Read the model definition and answer for the solid it produces. Units are mm, in the model's axes. A direction names the side the tool comes from. Coordinates: 2 decimals unless noted, no trailing zeros. Write each loop counter-clockwise with the first axis right and the second up, starting at its lowest first coordinate (ties: lowest second). Pieces come first, ordered by that corner, then holes. Notation, with made-up numbers: (80.5, 2.25) -> (87.5, 2.25) arc R35 ccw to (87.5, 36.25) -> close; hole circle Ø3 at (-10.5, 68). An arc over 180 degrees is marked (long way). Answer as a JSON object with one key per item and string values. Group by question number.
(1) Straight lines are drawn through the part: L1, parallel to Y at x = 0, z = 7.05; L2, parallel to X at y = 3, z = 6.75; L3, parallel to Z at x = 4.25, y = 3.75. For each, find the intervals that lie inside material, in ascending order.
(2) Find section D-D (z = 8.25). Give the vertices of the cut face in (x, y).
(3) Find section A-A (y = 0). Give the vertices of the cut face in (x, z).
(4) Find section C-C (z = 7.4). Give the vertices of the cut face in (x, y).
(5) Flat-ended cylindrical pins translate along their axes: P1, Ø2, axis at x = -4.33, y = 2.5, coming from the -Z side; P2, Ø1.8, axis at x = 0, y = 5, coming from the +Z side. Find the tip coordinate at first contact, or state that the pin passes through.
(6) Find section B-B (x = 0). Give the vertices of the cut face in (y, z).
(7) Which of the six approach directions +Z, -Z, +X, -X, +Y, -Y give full straight-line access (tool end or side, diameter ignored) to faces 4 (the face through (-0.878, -3.956, 8.364)), 5 (the face through (0.312, -5.597, 7.147))?
(8) For a pull along Y with two mould halves and no side action, classify faces 1 (the face through (2.805, -5.392, 7.013)), 2 (the face through (-1, 3, 9.182)), 3 (the face through (-3.684, 2.702, 7.147)) as +Y half, -Y half, draft (parallel to the pull), parting line (faces both ways), or undercut.
from build123d import *

# Parameters (mm, degrees)
SKETCH1_R           = 45
SKETCH1_R_2         = 30
SKETCH1_R_3         = 5
BOSS_EXTRUDE1_DEPTH = 10
SKETCH1_3_R         = 30
SKETCH1_3_R_2       = 20
BOSS_EXTRUDE2_DEPTH = 20
FILLET1_R           = 2
SCALE_1_SCALE       = 0.135064935


with BuildPart() as part:
    # Sketch1 → Boss-Extrude1 (new body)
    with BuildSketch(Plane.XY):
        Circle(SKETCH1_R)
        Circle(SKETCH1_R_2, mode=Mode.SUBTRACT)
        with Locations((-32.04293994, 18.5)):
            Circle(SKETCH1_R_3, mode=Mode.SUBTRACT)
        with Locations((-32.04293994, -18.5)):
            Circle(SKETCH1_R_3, mode=Mode.SUBTRACT)
        with Locations((0, -37)):
            Circle(SKETCH1_R_3, mode=Mode.SUBTRACT)
        with Locations((32.04293994, -18.5)):
            Circle(SKETCH1_R_3, mode=Mode.SUBTRACT)
        with Locations((32.04293994, 18.5)):
            Circle(SKETCH1_R_3, mode=Mode.SUBTRACT)
        with Locations((0, 37)):
            Circle(SKETCH1_R_3, mode=Mode.SUBTRACT)
    extrude(amount=BOSS_EXTRUDE1_DEPTH)

    # Sketch1_3 → Boss-Extrude2 (add)
    with BuildSketch(Plane.XY):
        Circle(SKETCH1_3_R)
        Circle(SKETCH1_3_R_2, mode=Mode.SUBTRACT)
    extrude(amount=BOSS_EXTRUDE2_DEPTH)

    # Fillet1
    fillet1_edges = [part.edges().sort_by_distance(p)[0] for p in [
        (-30, 0, 20),
        (-45, 0, 10),
    ]]
    fillet(fillet1_edges, radius=FILLET1_R)


with BuildPart() as part_1:
    # Scale 1: scaled about (0, 0, 7.492696154)
    add(part.part.scale(SCALE_1_SCALE).moved(Location((0, 0, 6.480695634))))


solid = part_1.part
Results below:
{
 "1": {"L1": "y = -6.08 to -5.67, -4.32 to -2.7, 2.7 to 4.32, 5.67 to 6.08", "L2": "x = -5.29 to -4.78, -3.88 to 3.88, 4.78 to 5.29", "L3": "z = 6.48 to 7.83"},
 "2": {"outline": "circle Ø8.1 at (0, 0); hole circle Ø5.4 at (0, 0)"},
 "3": {"outline": "(-6.08, 6.48) -> (-2.7, 6.48) -> (-2.7, 9.18) -> (-3.78, 9.18) arc R0.27 ccw to (-4.05, 8.91) -> (-4.05, 7.83) -> (-5.81, 7.83) arc R0.27 ccw to (-6.08, 7.56) -> close; (2.7, 6.48) -> (6.08, 6.48) -> (6.08, 7.56) arc R0.27 ccw to (5.81, 7.83) -> (4.05, 7.83) -> (4.05, 8.91) arc R0.27 ccw to (3.78, 9.18) -> (2.7, 9.18) -> close"},
 "4": {"outline": "circle Ø12.16 at (0, 0); hole circle Ø1.35 at (-4.33, -2.5); hole circle Ø1.35 at (-4.33, 2.5); hole circle Ø5.4 at (0, 0); hole circle Ø1.35 at (0, -5); hole circle Ø1.35 at (0, 5); hole circle Ø1.35 at (4.33, -2.5); hole circle Ø1.35 at (4.33, 2.5)"},
 "5": {"P1": "stops at z = 6.48", "P2": "stops at z = 7.83"},
 "6": {"outline": "(-6.08, 6.48) -> (-5.67, 6.48) -> (-5.67, 7.83) -> (-5.81, 7.83) arc R0.27 ccw to (-6.08, 7.56) -> close; (-4.32, 6.48) -> (-2.7, 6.48) -> (-2.7, 9.18) -> (-3.78, 9.18) arc R0.27 ccw to (-4.05, 8.91) -> (-4.05, 7.83) -> (-4.32, 7.83) -> close; (2.7, 6.48) -> (4.32, 6.48) -> (4.32, 7.83) -> (4.05, 7.83) -> (4.05, 8.91) arc R0.27 ccw to (3.78, 9.18) -> (2.7, 9.18) -> close; (5.67, 6.48) -> (6.08, 6.48) -> (6.08, 7.56) arc R0.27 ccw to (5.81, 7.83) -> (5.67, 7.83) -> close"},
 "7": {"face 4": "+Z", "face 5": "+Z, -Z"},
 "8": {"face 1": "parting line", "face 2": "draft", "face 3": "undercut"}
}
